Could you check a few things on this drawing? It's one solid part, dimensions in mm from its lowest x, y, z. A direction names the side the tool comes from. Round coordinates to 2 decimals unless told otherwise and drop trailing zeros. Loops run counter-clockwise (first coordinate to the right, second up) from the corner with the lowest first, then second, coordinate; pieces in that order, holes last. Notation, with made-up numbers: M 11.5,8 L 66.5,8 A30 cw 66.5,43 Z; hole C -15.5,56 d1. An arc over 180 degrees is marked long. Answer as a JSON object with one key per item and string values.
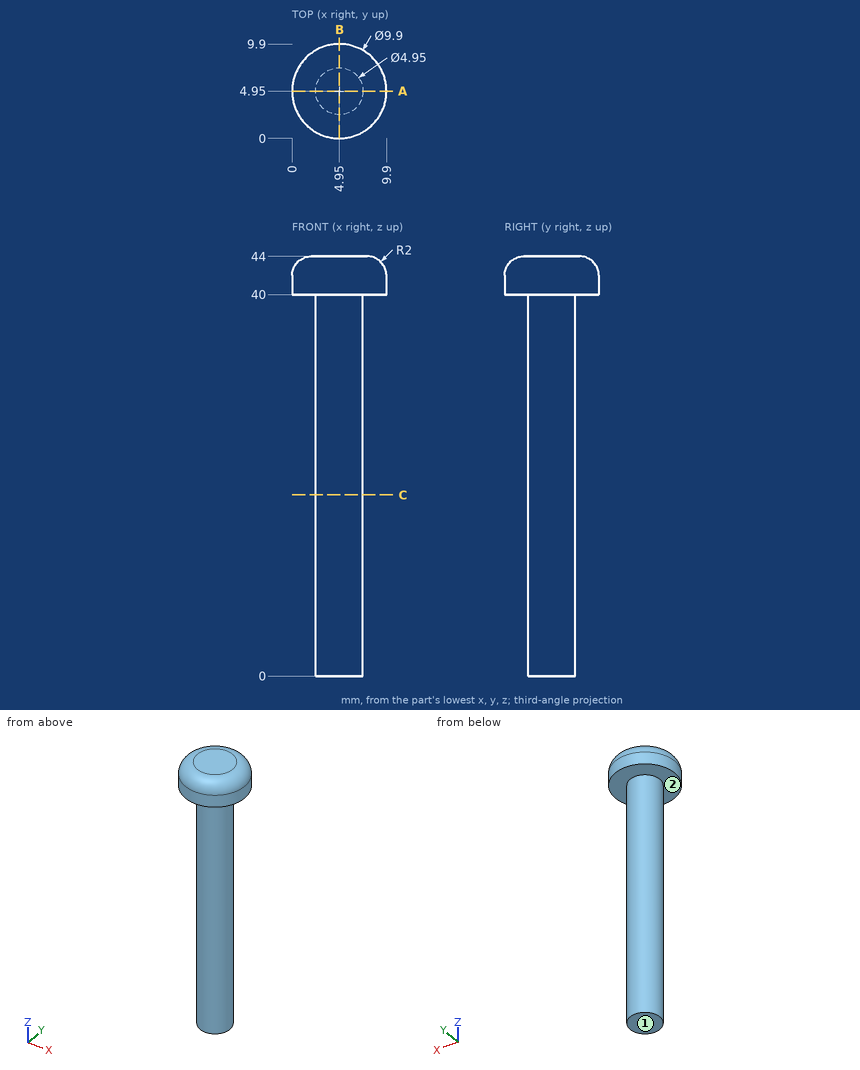
Item 1: I'm going to push flat-ended pins straight in: pin 1 Ø3 at (x, z) = (5.5, 15.5) entering from +Y (3 decimals); pin 2 Ø1.5 at (x, y) = (8.5, 2) entering from -Z; pin 3 Ø2 at (x, z) = (5.5, 22.5) entering from -Y (3 decimals). Where does each tip first touch, or does it pass through?
Resolved:
{"pin 1": "y = 7.425", "pin 2": "z = 40", "pin 3": "y = 2.475"}
Item 2: I want a section at C-C, the plane z = 19. Please give me the cut outline in (x, y) (3 decimals).
Resolved:
{"outline": "C 4.95,4.95 d4.95"}
Item 3: On a 3-axis mill with a long thin cutter (end or side, diameter ignored), from which of +Z, -Z, +X, -X, +Y, -Y can I reach the whole of each face in a straight line? I mean the marked faces 1 and 2. Say none if no direction works.
Resolved:
{"face 1": "-Z, +X, -X, +Y, -Y", "face 2": "-Z"}
Item 4: Please list where these lines run through material, in increasing order: probe 1 along Y at (x, z) = (5, 32); probe 2 along Y at (x, z) = (7.25, 41.5). Write a range as from..to.
Resolved:
{"probe 1": "2.48..7.42", "probe 2": "0.57..9.33"}
Item 5: I want a section at A-A, the plane y = 4.95. Please give me the cut outline in (x, z) (3 decimals), then the cut area to 3 significant figures.
Resolved:
{"outline": "M 0,40 L 2.475,40 L 2.475,0 L 7.425,0 L 7.425,40 L 9.9,40 L 9.9,42 A2 ccw 7.9,44 L 2,44 A2 ccw 0,42 Z", "area": "236 mm²"}
